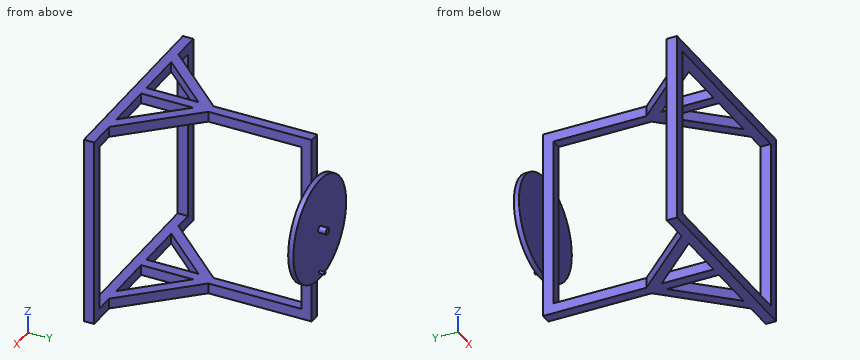
from build123d import *

# Parameters (mm, degrees)
BOSS_EXTRUDE1_DEPTH  = 740
SKETCH2_W            = 720
SKETCH2_H            = 660
CUT_EXTRUDE1_DEPTH   = 760
SKETCH4_W            = 25
SKETCH4_H            = 40
CUT_EXTRUDE2_DEPTH   = 817
SKETCH5_W            = 40
SKETCH5_H            = 40
BOSS_EXTRUDE2_DEPTH  = 740
SKETCH6_W            = 40
SKETCH6_H            = 40
BOSS_EXTRUDE3_DEPTH  = 740
SKETCH7_R            = 200
BOSS_EXTRUDE5_DEPTH  = 20
SKETCH8_R            = 12.5
BOSS_EXTRUDE6_DEPTH  = 30
SKETCH9_R            = 5
BOSS_EXTRUDE10_DEPTH = 20


with BuildPart() as part:
    # Sketch1 → Boss-Extrude1 (new body)
    with BuildSketch(Plane.XY):
        Polygon((-79.470198675, 173.509933775), (-79.470198675, -226.490066225), (-322.136865342, -486.490066225), (-459.470198675, -486.490066225), (-459.470198675, -526.490066225), (340.529801325, -526.490066225), (340.529801325, -486.490066225), (203.196467991, -486.490066225), (-39.470198675, -226.490066225), (-39.470198675, 173.509933775), align=None)
        Polygon((-79.470198675, -486.490066225), (-267.421439932, -486.490066225), (-79.470198675, -285.113736307), align=None, mode=Mode.SUBTRACT)
        Polygon((148.481042581, -486.490066225), (-39.470198675, -486.490066225), (-39.470198675, -285.113736307), align=None, mode=Mode.SUBTRACT)
    extrude(amount=BOSS_EXTRUDE1_DEPTH)

    # Sketch2 → Cut-Extrude1 (cut)
    with BuildSketch(Plane.XZ.offset(526.490066225)):
        with Locations((-59.470198675, 370)):
            Rectangle(SKETCH2_W, SKETCH2_H)
    extrude(amount=-CUT_EXTRUDE1_DEPTH, mode=Mode.SUBTRACT)

    # Sketch4 → Cut-Extrude2 (cut)
    with BuildSketch(Plane(origin=(0, 0, 0), x_dir=(-1, 0, 0), z_dir=(0, 0, -1))):
        with Locations((-328.029801325, -506.490066225)):
            Rectangle(SKETCH4_W, SKETCH4_H)
        with Locations((446.970198675, -506.490066225)):
            Rectangle(SKETCH4_W, SKETCH4_H)
    extrude(amount=-CUT_EXTRUDE2_DEPTH, mode=Mode.SUBTRACT)

    # Sketch5 → Boss-Extrude2 (add)
    with BuildSketch(Plane(origin=(0, 0, 0), x_dir=(-1, 0, 0), z_dir=(0, 0, -1))):
        with Locations((-295.529801325, -506.490066225)):
            Rectangle(SKETCH5_W, SKETCH5_H)
        with Locations((414.470198675, -506.490066225)):
            Rectangle(SKETCH5_W, SKETCH5_H)
    extrude(amount=-BOSS_EXTRUDE2_DEPTH)

    # Sketch6 → Boss-Extrude3 (add)
    with BuildSketch(Plane(origin=(0, 0, 0), x_dir=(-1, 0, 0), z_dir=(0, 0, -1))):
        with Locations((59.470198675, 153.509933775)):
            Rectangle(SKETCH6_W, SKETCH6_H)
    extrude(amount=-BOSS_EXTRUDE3_DEPTH)

    # Sketch7 → Boss-Extrude5 (add)
    with BuildSketch(Plane(origin=(0, 173.509933775, 0), x_dir=(1, 0, 0), z_dir=(0, 1, 0))):
        with Locations((-61.40332894, -370)):
            Circle(SKETCH7_R)
    extrude(amount=BOSS_EXTRUDE5_DEPTH)

    # Sketch8 → Boss-Extrude6 (add)
    with BuildSketch(Plane(origin=(0, 193.509933775, 0), x_dir=(1, 0, 0), z_dir=(0, 1, 0))):
        with Locations((-61.40332894, -370)):
            Circle(SKETCH8_R)
    extrude(amount=BOSS_EXTRUDE6_DEPTH)

    # Sketch9 → Boss-Extrude10 (add)
    with BuildSketch(Plane(origin=(0, 193.509933775, 0), x_dir=(1, 0, 0), z_dir=(0, 1, 0))):
        with Locations((-59.876755941, -196.697911229)):
            Circle(SKETCH9_R)
    extrude(amount=BOSS_EXTRUDE10_DEPTH)


solid = part.part
Work out the finished part from the listing and answer in its coordinate system (mm). Give positions to 0.01 mm unless a question says otherwise; leave off trailing zeros. Order: outer loops, then holes, each group sorted by start corner. A loop starts at its lowest first (then second) coordinate and runs counter-clockwise, first axis right, second up. Notation, with made-up numbers: (22, 65.5) -> (34, 65.5) arc R19 ccw to (34, 96.5) -> close; hole circle Ø10 at (40.25, 80). An arc over 180 degrees is marked (long way). Answer as a JSON object with one key per item and string values. Group by question number.
1. Consider line 1 along Z through (x, y) = (134, -414.5); line 2 along X through (y, z) = (-366, 710); line 3 along Y through (x, z) = (40.5, 462). Determine where each line is inside the solid, lowest interval first. Write a range as [from, to].
2. Flat-ended cylindrical pins translate along their axes: pin 1 Ø2 at (x, z) = (47.5, 446.5) entering from -Y; pin 2 Ø20 at (y, z) = (-343, 729) entering from +X; pin 3 Ø11 at (x, z) = (-61, 198.5) entering from +Y. Find the tip coordinate at first contact, or state that the pin passes through.
3. Section C-C on x = -371 is taken. Determine the outline of the cut face in (y, z).
4. Section A-A on z = 370 is taken. Determine the outline of the cut face in (x, y).
5. Section D-D on y = -389.5 is taken. Determine the outline of the cut face in (x, z), plus the area to 3 significant figures.
6. Section B-B on y = -63 is taken. Determine the outline of the cut face in (x, z), plus the area to 3 significant figures.
Result sheet:
{
 "1": {"line 1": "z = [0, 40], [700, 740]", "line 2": "x = [-209.68, -154.96], [-79.47, -39.47], [36.02, 90.74]", "line 3": "y = [173.51, 193.51]"},
 "2": {"pin 1": "stops at y = 173.51", "pin 2": "stops at x = 78.61", "pin 3": "stops at y = 213.51"},
 "3": {"outline": "(-526.49, 0) -> (-486.49, 0) -> (-486.49, 40) -> (-526.49, 40) -> close; (-526.49, 700) -> (-486.49, 700) -> (-486.49, 740) -> (-526.49, 740) -> close"},
 "4": {"outline": "(-434.47, -526.49) -> (-394.47, -526.49) -> (-394.47, -486.49) -> (-434.47, -486.49) -> close; (-261.4, 173.51) -> (-79.47, 173.51) -> (-79.47, 133.51) -> (-39.47, 133.51) -> (-39.47, 173.51) -> (138.6, 173.51) -> (138.6, 193.51) -> (-48.9, 193.51) -> (-48.9, 223.51) -> (-73.9, 223.51) -> (-73.9, 193.51) -> (-261.4, 193.51) -> close; (275.53, -526.49) -> (315.53, -526.49) -> (315.53, -486.49) -> (275.53, -486.49) -> close"},
 "5": {"outline": "(-231.61, 0) -> (-176.9, 0) -> (-176.9, 40) -> (-231.61, 40) -> close; (-231.61, 700) -> (-176.9, 700) -> (-176.9, 740) -> (-231.61, 740) -> close; (-79.47, 0) -> (-39.47, 0) -> (-39.47, 40) -> (-79.47, 40) -> close; (-79.47, 700) -> (-39.47, 700) -> (-39.47, 740) -> (-79.47, 740) -> close; (57.96, 0) -> (112.67, 0) -> (112.67, 40) -> (57.96, 40) -> close; (57.96, 700) -> (112.67, 700) -> (112.67, 740) -> (57.96, 740) -> close", "area": "12,000 mm^2"},
 "6": {"outline": "(-79.47, 0) -> (-39.47, 0) -> (-39.47, 40) -> (-79.47, 40) -> close; (-79.47, 700) -> (-39.47, 700) -> (-39.47, 740) -> (-79.47, 740) -> close", "area": "3,200 mm^2"}
}
